Geometry: final body of the model. Coordinates: model frame, mm. Face numbers are marked on the shaded views. Give positions to 0.01 mm unless a question says otherwise; leave off trailing zeros. Loops run counter-clockwise (first coordinate to the right, second up) from the corner with the lowest first, then second, coordinate; pieces in that order, holes last. Notation, with made-up numbers: M 36.25,-40 L 59.25,-40 A28 ccw 59.25,-12 Z; hole C 45.25,-3.75 d2. An arc over 180 degrees is marked long. One line per question, with ' | ' between items. Start each with the question number.
Autodesk Fusion 360 part; units mm, degrees
sketch "Sketch1" plane through (0, 0, 0) normal (0, 0, 1) x (1, 0, 0)
  line L0 (-14.75, -2.5675) -> (-10.6089, -2.5675)
  line L1 (-10.6089, -2.5675) -> (-10.6082, -2.5702)
  line L2 (-10.6404, 2.5117) -> (-14.7873, 2.5117)
  arc A0 (-14.75, -2.5675) -> (-14.7873, 2.5117) centre (-0.0603, 0.0802) ccw
  arc A1 (-12.8266, -2.5675) -> (-12.8696, 2.5117) centre (-0.0603, 0.0802) ccw
  arc A2 (-10.6082, -2.5702) -> (-10.6589, 2.5117) centre (-0.0605, 0.0763) ccw
sketch "Sketch3" plane through (0, 0, 0) normal (0, 0, 1) x (1, 0, 0)
extrude "Extrude1" add sketch "Sketch1" along normal blind 6.35 contours L0 L2 A0 A1
extrude "Extrude4" cut sketch "Sketch1" along normal blind 43.18 contours L0 L1 L2 A1 A2
extrude "Extrude5" add sketch "Sketch1" along normal blind 50.8 contours L0 L1 L2 A1 A2
extrude "Extrude3" [suppressed]
extrude "Extrude2" [suppressed]
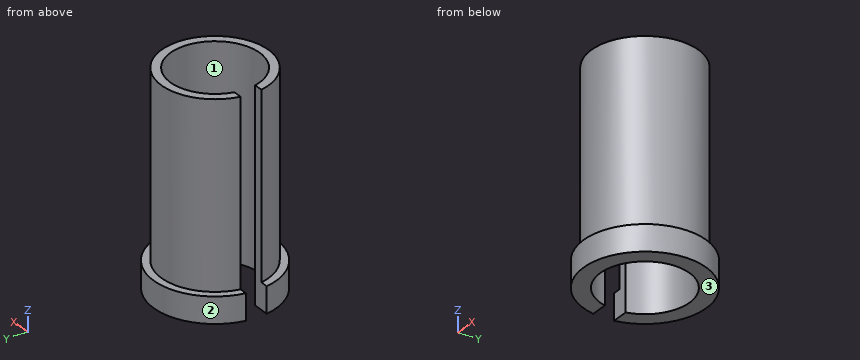
Q1. Section D-D, the plane y = 0.75. Output: boundary loops of the cut face in (x, z).
Q2. Contact query for flat-ended pins moving along their axis: pin 1 (8 mm diameter, centred on x = 11.5, z = 19.5, fed in from +Y); pin 2 (5 mm diameter, centred on x = 1.5, z = 33, fed in from -Y); pin 3 (4 mm diameter, centred on x = 8, z = 32.5, fed in from -Y); pin 4 (13 mm diameter, centred on x = -0.06, y = 0.08, fed in from -Z). Output: stop coordinate, or through.
Q3. Draft query along Y for the marked faces 1, 2 and 3. Return one class per face: released by +Y, released by -Y, zero draft, split by the parting line, or undercut.
Q4. Section B-B, the plane x = 1.75. Output: boundary loops of the cut face in (y, z).
Q5. Section A-A, the plane y = -8. Output: boundary loops of the cut face in (x, z).
Q6. Material intervals for L1, parallel to Y at x = -0.5, z = 30; L2, parallel to Z at x = 12.75, y = -6.25; L3, parallel to X at y = 4.5, z = 12.5, sorted ascending.
Model answer:
1) outline: M 10.79,0 L 14.85,0 L 14.85,6.35 L 12.96,6.35 L 12.96,50.8 L 10.79,50.8 Z
2) pin 1: stops at y = 10.7 | pin 2: stops at y = -12.96 | pin 3: stops at y = -11.46 | pin 4: passes through
3) face 1: undercut | face 2: split by the parting line | face 3: zero draft
4) outline: M -14.74,0 L -10.65,0 L -10.65,50.8 L -12.83,50.8 L -12.83,6.35 L -14.74,6.35 Z; M 10.8,0 L 14.9,0 L 14.9,6.35 L 12.99,6.35 L 12.99,50.8 L 10.8,50.8 Z
5) outline: M -12.61,0 L -7.34,0 L -7.34,50.8 L -10.29,50.8 L -10.29,6.35 L -12.61,6.35 Z; M 7.22,0 L 12.49,0 L 12.49,6.35 L 10.17,6.35 L 10.17,50.8 L 7.22,50.8 Z
6) L1: y = -12.95 to -10.79, 10.94 to 13.11 | L2: z = 0 to 6.35 | L3: x = -12.33 to -9.99, 9.87 to 12.21
